from build123d import *

# Parameters (mm, degrees)
F0_W     = 40.1
F0_H     = 78.2
F0_W_2   = 38.1
F0_H_2   = 76.2
F1_DEPTH = 6.35
F2_W     = 40.1
F2_H     = 78.2
F2_W_2   = 38.1
F2_H_2   = 76.2
F3_DEPTH = 57.15
F4_SIZE2 = 3.17499
F4_SIZE  = 0.49999
F5_R     = 1.27


# Not quite as in the source:
# - a fillet or chamfer is up to 0.001 mm smaller than in the source, because OpenCascade refuses the exact size


with BuildPart() as f1:
    # F0 (on Top) → F1 (new body)
    with BuildSketch(Plane.XY):
        with BuildLine():
            ThreePointArc((25.4, 38.1), (23.5401280605, 42.5901280605), (19.05, 44.45))
            Line((19.05, 44.45), (-19.05, 44.45))
            ThreePointArc((-19.05, 44.45), (-23.5401280605, 42.5901280605), (-25.4, 38.1))
            Line((-25.4, 38.1), (-25.4, -38.1))
            ThreePointArc((-25.4, -38.1), (-23.5401280605, -42.5901280605), (-19.05, -44.45))
            Line((-19.05, -44.45), (19.05, -44.45))
            ThreePointArc((19.05, -44.45), (23.5401280605, -42.5901280605), (25.4, -38.1))
            Line((25.4, -38.1), (25.4, 38.1))
        make_face()
        Rectangle(F0_W, F0_H, mode=Mode.SUBTRACT)
        Rectangle(F0_W, F0_H)
        Rectangle(F0_W_2, F0_H_2, mode=Mode.SUBTRACT)
    extrude(amount=F1_DEPTH)

    # F2 (on face) → F3 (join)
    with BuildSketch(Plane(origin=(0, 0, 0), x_dir=(1, 0, 0), z_dir=(0, 0, -1))):
        Rectangle(F2_W, F2_H)
        Rectangle(F2_W_2, F2_H_2, mode=Mode.SUBTRACT)
    extrude(amount=F3_DEPTH)

    # F4 (size 0.5 and 3.175 in the source; OpenCascade refuses exactly that, so slightly less here)
    f4_edges = [f1.edges().sort_by_distance(p)[0] for p in [
        (-20.05, 0, -57.15),
        (0, 39.1, -57.15),
        (20.05, 0, -57.15),
        (0, -39.1, -57.15),
        (0, -38.1, -57.15),
        (19.05, 0, -57.15),
        (0, 38.1, -57.15),
        (-19.05, 0, -57.15),
    ]]
    f4_side = f1.faces().sort_by_distance((-19.17118, 0, -57.15))[0]
    chamfer(f4_edges, length=F4_SIZE, length2=F4_SIZE2, reference=f4_side)

    # F5
    f5_edges = [f1.edges().sort_by_distance(p)[0] for p in [
        (23.540128, 42.590128, 6.35),
        (0, 44.45, 6.35),
        (-23.540128, 42.590128, 6.35),
        (-25.4, 0, 6.35),
        (-23.540128, -42.590128, 6.35),
        (0, -44.45, 6.35),
        (23.540128, -42.590128, 6.35),
        (25.4, 0, 6.35),
        (0, -38.1, 6.35),
        (-19.05, 0, 6.35),
        (0, 38.1, 6.35),
        (19.05, 0, 6.35),
    ]]
    fillet(f5_edges, radius=F5_R)


solid = f1.part
For this review, take the finished solid that the model builds, in its own axes (mm). A direction names the side the tool comes from. Give positions to 0.01 mm unless a question says otherwise; leave off trailing zeros. Order: outer loops, then holes, each group sorted by start corner. A loop starts at its lowest first (then second) coordinate and runs counter-clockwise, first axis right, second up. Notation, with made-up numbers: (16.5, 20) -> (75.5, 20) arc R22 cw to (75.5, 30) -> close; hole circle Ø10 at (35.5, 87). An arc over 180 degrees is marked (long way). Write item = value, one per line.
1) Draft analysis for pull direction X (two halves, no side actions). For faces 1 (the face through (-23.59, -42.54, 2.5)), 2 (the face through (-0.281, 38.854, -55.54)), 3 (the face through (0, 38.1, -24)), 4 (the face through (19.296, 0.54, -55.54)), state which applies: pulls with the +X half, pulls with the -X half, needs draft (parallel to the pull), parting line crosses it, or undercut.
Findings:
face_1 = pulls with the -X half
face_2 = needs draft
face_3 = undercut
face_4 = undercut
2) We need section C-C, the plane z = -16.5. Give the boundary of the cut face in (x, y).
Findings:
outline = (-20.05, -39.1) -> (20.05, -39.1) -> (20.05, 39.1) -> (-20.05, 39.1) -> close; hole (-19.05, -38.1) -> (19.05, -38.1) -> (19.05, 38.1) -> (-19.05, 38.1) -> close
3) To check wall thickness, follow L1, parallel to Y at x = -7, z = -43; L2, parallel to X at y = 17, z = -13; L3, parallel to Z at x = 21, y = 6.5. State the ranges of each line that lie inside material, in increasing order. Write a range as from..to.
Findings:
L1 = -39.1..-38.1, 38.1..39.1
L2 = -20.05..-19.05, 19.05..20.05
L3 = 0..6.35
4) Insertion check: pin 1 (20 mm diameter, centred on x = 9, z = -28.5, fed in from +Y); pin 2 (19 mm diameter, centred on x = -4, z = -29, fed in from -Y); pin 3 (17.5 mm diameter, centred on y = -10, z = -26.5, fed in from -X). Each pin has a flat end and moves straight along its axis. Give the tip position at first contact, or say it passes through.
Findings:
pin_1 = 39.1
pin_2 = -39.1
pin_3 = -20.05
5) For faces 5 (the face through (-0.274, -38.346, -55.54)), 6 (the face through (-19.05, 1, -24)), 7 (the face through (0, -39.1, -27)), list the 3-axis set-ups (+Z, -Z, +X, -X, +Y, -Y) from which the entire face can be reached by the end or side of a thin tool; tool diameter is ignored.
Findings:
face_5 = -Z
face_6 = +Z, -Z
face_7 = -Z, +X, -X, -Y
